Geometry: final body of the model. Coordinates: model frame, mm. A direction names the side the tool comes from. Give positions to 0.01 mm unless a question says otherwise; leave off trailing zeros. Write each loop counter-clockwise with the first axis right and the second up, starting at its lowest first coordinate (ties: lowest second). Pieces come first, ordered by that corner, then holes. Notation, with made-up numbers: (9.5, -22) -> (39.5, -22) arc R17 ccw to (39.5, 2) -> close; hole circle Ø10 at (-13.75, -39.75). An arc over 180 degrees is marked (long way). Answer as a JSON object with one key per item and string values.
from build123d import *

# Parameters (mm, degrees)
F0_W     = 12.7
F0_H     = 25.4
F1_DEPTH = 6.35
F2_R     = 6.34999


# Not quite as in the source:
# - a fillet or chamfer is up to 0.001 mm smaller than in the source, because OpenCascade refuses the exact size


with BuildPart() as f1:
    # F0 (on Top) → F1 (new body, symmetric)
    with BuildSketch(Plane.XY):
        Polygon((6.35, 0), (-6.35, 0), (-24.3105122421, -17.9605122421), (-15.3302561211, -26.9407683632), (0, -11.6105122421), (15.3302561211, -26.9407683632), (24.3105122421, -17.9605122421), align=None)
        with Locations((0, 12.7)):
            Rectangle(F0_W, F0_H)
    extrude(amount=F1_DEPTH, both=True)

    # F2 (radius 6.35 in the source; OpenCascade refuses exactly that, so slightly less here)
    f2_edges = [f1.edges().sort_by_distance(p)[0] for p in [
        (6.35, 12.7, 6.35),
        (6.35, 12.7, -6.35),
        (-6.35, 12.7, 6.35),
        (-6.35, 12.7, -6.35),
        (15.330256, -8.980256, 6.35),
        (15.330256, -8.980256, -6.35),
        (7.665128, -19.27564, 6.35),
        (7.665128, -19.27564, -6.35),
        (-7.665128, -19.27564, 6.35),
        (-7.665128, -19.27564, -6.35),
        (-15.330256, -8.980256, 6.35),
        (-15.330256, -8.980256, -6.35),
    ]]
    fillet(f2_edges, radius=F2_R)


solid = f1.part
Q1. Mould query, pull axis X, two halves, no side actions, for faces 5 (the cylindrical face through (-13.26, -9.47, -4.44)), 6 (the cylindrical face through (9.04, -18.09, -4.44)), 7 (the cylindrical face through (9.04, -18.09, 4.44)), 8 (the flat face through (19.76, -22.51, 0.09)). Classes: pulls with the +X half, pulls with the -X half, needs draft (parallel to the pull), parting line crosses it, or undercut.
Values:
{"face 5": "pulls with the -X half", "face 6": "undercut", "face 7": "undercut", "face 8": "pulls with the +X half"}
Q2. Material intervals for L1, parallel to Z at x = -17.5, y = -20.5; L2, parallel to Y at x = 8.5, z = 1.75; L3, parallel to X at y = 23, z = 1, sorted ascending. Write a range as from..to.
Values:
{"L1": "-6.34..6.34", "L2": "-19.76..-2.5", "L3": "-6.27..6.27"}
Q3. First-contact query: P1, Ø1, axis at x = -6, y = 10, coming from the +Z side; P2, Ø2, axis at y = -2, z = 5, coming from the -X side; P3, Ø1, axis at x = -16, z = 1.5, coming from the -Y side. Flat tips, straight axial feed; report the tip coordinate or a pass-through.
Values:
{"P1": "z = 3.17", "P2": "x = -6.71", "P3": "y = -26.77"}
Q4. Cut plane B-B (z = 2.5). Return the cut outline in (x, y).
Values:
{"outline": "(-23.95, -18.32) -> (-15.69, -26.58) -> (0, -10.89) -> (15.69, -26.58) -> (23.95, -18.32) -> (5.84, -0.21) -> (5.84, 25.4) -> (-5.84, 25.4) -> (-5.84, -0.21) -> close"}
Q5. Cut plane C-C (z = -3). Return the cut outline in (x, y), and give its area (3 significant figures).
Values:
{"outline": "(-23.78, -18.49) -> (-15.86, -26.41) -> (0, -10.55) -> (15.86, -26.41) -> (23.78, -18.49) -> (5.6, -0.31) -> (5.6, 25.4) -> (-5.6, 25.4) -> (-5.6, -0.31) -> close", "area": "884 mm²"}
Q6. Set-up query: faces 1 (the cylindrical face through (-8.76, -17.81, -4.44)), 2 (the cylindrical face through (4.54, 11.58, -4.44)), 3 (the cylindrical face through (-8.76, -17.81, 4.44)), 4 (the cylindrical face through (-4.54, 11.58, -4.44)). Return all of +Z, -Z, +X, -X, +Y, -Y with unobstructed straight access to the full face (end or side cutting, diameter ignored); none if empty.
Values:
{"face 1": "-Z, -Y", "face 2": "-Z, +X, +Y", "face 3": "+Z, -Y", "face 4": "-Z, -X, +Y"}
